Model file for the job. Use its own axes, mm. Round coordinates to 2 decimals unless told otherwise and drop trailing zeros. Loops run counter-clockwise (first coordinate to the right, second up) from the corner with the lowest first, then second, coordinate; pieces in that order, holes last. Notation, with made-up numbers: (33, -18) -> (50, -18) arc R26 ccw to (50, 9) -> close; hole circle Ø10 at (38, 4). An arc over 180 degrees is marked (long way). Use a Markdown table: item, result. Add a question column.
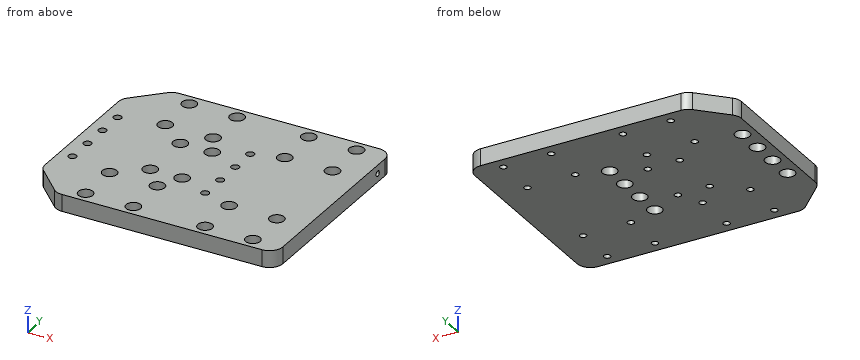
```python
from build123d import *

# Parameters (mm, degrees)
SKETCH1_R                 = 2.5
BOSS_EXTRUDE1_DEPTH       = 12.7
SKETCH2_R                 = 5.5
CUT_EXTRUDE1_DEPTH        = 7
CUT_EXTRUDE2_REACH        = 133.416
SKETCH3_R                 = 3
SKETCH4_R                 = 5.5
CUT_EXTRUDE3_DEPTH        = 7
CHAMFER1_SIZE             = 25
FILLET1_R                 = 10
M5X0_8_TAPPED_HOLE1_D     = 4.2
M5X0_8_TAPPED_HOLE1_DEPTH = 19
M5X0_8_TAPPED_HOLE1_TIP   = 1.2618073


with BuildPart() as part:
    # Sketch1 → Boss-Extrude1 (new body)
    with BuildSketch(Plane.XY):
        Polygon((-85, 78), (85, 78), (85, -78), (-85, -78), (-105, -78), (-105, 78), align=None)
        with Locations((27, -37)):
            Circle(SKETCH1_R, mode=Mode.SUBTRACT)
        with Locations((63, -37)):
            Circle(SKETCH1_R, mode=Mode.SUBTRACT)
        with Locations((27, -69)):
            Circle(SKETCH1_R, mode=Mode.SUBTRACT)
        with Locations((63, -69)):
            Circle(SKETCH1_R, mode=Mode.SUBTRACT)
        with Locations(Location((-63, -37, 0), (0, 0, 180))):
            Circle(SKETCH1_R, mode=Mode.SUBTRACT)
        with Locations(Location((-63, -69, 0), (0, 0, 180))):
            Circle(SKETCH1_R, mode=Mode.SUBTRACT)
        with Locations(Location((-27, -69, 0), (0, 0, 180))):
            Circle(SKETCH1_R, mode=Mode.SUBTRACT)
        with Locations(Location((-27, -37, 0), (0, 0, 180))):
            Circle(SKETCH1_R, mode=Mode.SUBTRACT)
        with Locations(Location((63, 69, 0), (0, 0, 180))):
            Circle(SKETCH1_R, mode=Mode.SUBTRACT)
        with Locations(Location((63, 37, 0), (0, 0, 180))):
            Circle(SKETCH1_R, mode=Mode.SUBTRACT)
        with Locations(Location((27, 69, 0), (0, 0, 180))):
            Circle(SKETCH1_R, mode=Mode.SUBTRACT)
        with Locations(Location((27, 37, 0), (0, 0, 180))):
            Circle(SKETCH1_R, mode=Mode.SUBTRACT)
        with Locations((-27, 69)):
            Circle(SKETCH1_R, mode=Mode.SUBTRACT)
        with Locations((-27, 37)):
            Circle(SKETCH1_R, mode=Mode.SUBTRACT)
        with Locations((-63, 69)):
            Circle(SKETCH1_R, mode=Mode.SUBTRACT)
        with Locations((-63, 37)):
            Circle(SKETCH1_R, mode=Mode.SUBTRACT)
        with Locations((-42, 20)):
            Circle(SKETCH1_R, mode=Mode.SUBTRACT)
        with Locations((-18, 20)):
            Circle(SKETCH1_R, mode=Mode.SUBTRACT)
        with Locations((-42, -20)):
            Circle(SKETCH1_R, mode=Mode.SUBTRACT)
        with Locations((-18, -20)):
            Circle(SKETCH1_R, mode=Mode.SUBTRACT)
    extrude(amount=BOSS_EXTRUDE1_DEPTH)

    # Sketch2 → Cut-Extrude1 (cut)
    with BuildSketch(Plane.XY.offset(12.7)):
        with Locations((-63, 69)):
            Circle(SKETCH2_R)
        with Locations((-27, 69)):
            Circle(SKETCH2_R)
        with Locations((-63, 37)):
            Circle(SKETCH2_R)
        with Locations((-27, 37)):
            Circle(SKETCH2_R)
        with Locations((27, 69)):
            Circle(SKETCH2_R)
        with Locations((63, 69)):
            Circle(SKETCH2_R)
        with Locations((27, 37)):
            Circle(SKETCH2_R)
        with Locations((63, 37)):
            Circle(SKETCH2_R)
        with Locations((-42, 20)):
            Circle(SKETCH2_R)
        with Locations((-18, 20)):
            Circle(SKETCH2_R)
        with Locations((-42, -20)):
            Circle(SKETCH2_R)
        with Locations((-18, -20)):
            Circle(SKETCH2_R)
        with Locations((-63, -37)):
            Circle(SKETCH2_R)
        with Locations((-27, -37)):
            Circle(SKETCH2_R)
        with Locations((-63, -69)):
            Circle(SKETCH2_R)
        with Locations((-27, -69)):
            Circle(SKETCH2_R)
        with Locations((27, -69)):
            Circle(SKETCH2_R)
        with Locations((27, -37)):
            Circle(SKETCH2_R)
        with Locations((63, -37)):
            Circle(SKETCH2_R)
        with Locations((63, -69)):
            Circle(SKETCH2_R)
    extrude(amount=-CUT_EXTRUDE1_DEPTH, mode=Mode.SUBTRACT)

    # Sketch3 → Cut-Extrude2 (cut, up to next)
    with BuildSketch(Plane.XY.offset(12.7), mode=Mode.PRIVATE) as cut_extrude2_sk1:
        with Locations((-95, 30)):
            Circle(SKETCH3_R)
    cut_extrude2_tool1 = extrude(cut_extrude2_sk1.sketch, amount=-CUT_EXTRUDE2_REACH, mode=Mode.PRIVATE) & part.part
    # Sketch3 → Cut-Extrude2 (cut, up to next)
    with BuildSketch(Plane.XY.offset(12.7), mode=Mode.PRIVATE) as cut_extrude2_sk2:
        with Locations((-95, 10)):
            Circle(SKETCH3_R)
    cut_extrude2_tool2 = extrude(cut_extrude2_sk2.sketch, amount=-CUT_EXTRUDE2_REACH, mode=Mode.PRIVATE) & part.part
    # Sketch3 → Cut-Extrude2 (cut, up to next)
    with BuildSketch(Plane.XY.offset(12.7), mode=Mode.PRIVATE) as cut_extrude2_sk3:
        with Locations((-95, -10)):
            Circle(SKETCH3_R)
    cut_extrude2_tool3 = extrude(cut_extrude2_sk3.sketch, amount=-CUT_EXTRUDE2_REACH, mode=Mode.PRIVATE) & part.part
    # Sketch3 → Cut-Extrude2 (cut, up to next)
    with BuildSketch(Plane.XY.offset(12.7), mode=Mode.PRIVATE) as cut_extrude2_sk4:
        with Locations((-95, -30)):
            Circle(SKETCH3_R)
    cut_extrude2_tool4 = extrude(cut_extrude2_sk4.sketch, amount=-CUT_EXTRUDE2_REACH, mode=Mode.PRIVATE) & part.part
    # Sketch3 → Cut-Extrude2 (cut, up to next)
    with BuildSketch(Plane.XY.offset(12.7), mode=Mode.PRIVATE) as cut_extrude2_sk5:
        with Locations((5, -30)):
            Circle(SKETCH3_R)
    cut_extrude2_tool5 = extrude(cut_extrude2_sk5.sketch, amount=-CUT_EXTRUDE2_REACH, mode=Mode.PRIVATE) & part.part
    # Sketch3 → Cut-Extrude2 (cut, up to next)
    with BuildSketch(Plane.XY.offset(12.7), mode=Mode.PRIVATE) as cut_extrude2_sk6:
        with Locations((5, -10)):
            Circle(SKETCH3_R)
    cut_extrude2_tool6 = extrude(cut_extrude2_sk6.sketch, amount=-CUT_EXTRUDE2_REACH, mode=Mode.PRIVATE) & part.part
    # Sketch3 → Cut-Extrude2 (cut, up to next)
    with BuildSketch(Plane.XY.offset(12.7), mode=Mode.PRIVATE) as cut_extrude2_sk7:
        with Locations((5, 10)):
            Circle(SKETCH3_R)
    cut_extrude2_tool7 = extrude(cut_extrude2_sk7.sketch, amount=-CUT_EXTRUDE2_REACH, mode=Mode.PRIVATE) & part.part
    # Sketch3 → Cut-Extrude2 (cut, up to next)
    with BuildSketch(Plane.XY.offset(12.7), mode=Mode.PRIVATE) as cut_extrude2_sk8:
        with Locations((5, 30)):
            Circle(SKETCH3_R)
    cut_extrude2_tool8 = extrude(cut_extrude2_sk8.sketch, amount=-CUT_EXTRUDE2_REACH, mode=Mode.PRIVATE) & part.part
    add(cut_extrude2_tool1.solids().sort_by_distance((-95, 30, 12.7))[0], mode=Mode.SUBTRACT)
    add(cut_extrude2_tool2.solids().sort_by_distance((-95, 10, 12.7))[0], mode=Mode.SUBTRACT)
    add(cut_extrude2_tool3.solids().sort_by_distance((-95, -10, 12.7))[0], mode=Mode.SUBTRACT)
    add(cut_extrude2_tool4.solids().sort_by_distance((-95, -30, 12.7))[0], mode=Mode.SUBTRACT)
    add(cut_extrude2_tool5.solids().sort_by_distance((5, -30, 12.7))[0], mode=Mode.SUBTRACT)
    add(cut_extrude2_tool6.solids().sort_by_distance((5, -10, 12.7))[0], mode=Mode.SUBTRACT)
    add(cut_extrude2_tool7.solids().sort_by_distance((5, 10, 12.7))[0], mode=Mode.SUBTRACT)
    add(cut_extrude2_tool8.solids().sort_by_distance((5, 30, 12.7))[0], mode=Mode.SUBTRACT)

    # Sketch4 → Cut-Extrude3 (cut)
    with BuildSketch(Plane(origin=(0, 0, 0), x_dir=(-1, 0, 0), z_dir=(0, 0, -1))):
        with Locations((-5, 30)):
            Circle(SKETCH4_R)
        with Locations((-5, 10)):
            Circle(SKETCH4_R)
        with Locations((-5, -10)):
            Circle(SKETCH4_R)
        with Locations((-5, -30)):
            Circle(SKETCH4_R)
        with Locations((95, 30)):
            Circle(SKETCH4_R)
        with Locations((95, 10)):
            Circle(SKETCH4_R)
        with Locations((95, -10)):
            Circle(SKETCH4_R)
        with Locations((95, -30)):
            Circle(SKETCH4_R)
    extrude(amount=-CUT_EXTRUDE3_DEPTH, mode=Mode.SUBTRACT)

    # Chamfer1
    chamfer1_edges = [part.edges().sort_by_distance(p)[0] for p in [
        (-105, -78, 6.35),
        (-105, 78, 6.35),
    ]]
    chamfer(chamfer1_edges, length=CHAMFER1_SIZE)

    # Fillet1
    fillet1_edges = [part.edges().sort_by_distance(p)[0] for p in [
        (85, 78, 6.35),
        (85, -78, 6.35),
        (-105, -53, 6.35),
        (-105, 53, 6.35),
        (-80, 78, 6.35),
        (-80, -78, 6.35),
    ]]
    fillet(fillet1_edges, radius=FILLET1_R)

    # M5x0.8 Tapped Hole1
    with Locations(Plane(origin=(85, 0, 0), x_dir=(0, 0, -1), z_dir=(1, 0, 0))):
        with Locations((-6.35, 58.25)):
            Hole(M5X0_8_TAPPED_HOLE1_D / 2, depth=M5X0_8_TAPPED_HOLE1_DEPTH)
            with Locations((0, 0, -(M5X0_8_TAPPED_HOLE1_DEPTH + M5X0_8_TAPPED_HOLE1_TIP / 2))):  # 118° drill point
                Cone(0, M5X0_8_TAPPED_HOLE1_D / 2, M5X0_8_TAPPED_HOLE1_TIP, mode=Mode.SUBTRACT)


solid = part.part
```
1) Pin check, flat tips, straight feed: pin 1 Ø6.5 at (y, z) = (58.25, 6.35) entering from -X; pin 2 Ø5.5 at (x, y) = (-63.5, 68) entering from +Z; pin 3 Ø5 at (x, z) = (-78.5, 6.5) entering from -Y. Stop position of each tip, or through.
2) Cut at B-B on y = 20. Write the cut outline in (x, z).
3) Wall check: probe 1 along Y at (x, z) = (-63, 4.15); probe 2 along X at (y, z) = (37, 2); probe 3 along Y at (x, z) = (-18, 10). Give the ranges that are in metal, low to high. Write a range as from..to.
4) Cut at C-C on x = 5. Count the separate pieces of the cut face and the enclosed holes in it, and give its area (3 significant figures).
5) Cut at A-A on x = -42. Write the cut outline in (y, z).
Established:
| question | item | result |
|---|---|---|
| 1 | pin 1 | stops at x = -102.89 |
| 1 | pin 2 | stops at z = 5.7 |
| 1 | pin 3 | stops at y = -78 |
| 2 | outline | (-105, 0) -> (-44.5, 0) -> (-44.5, 5.7) -> (-47.5, 5.7) -> (-47.5, 12.7) -> (-105, 12.7) -> close; (-39.5, 0) -> (-20.5, 0) -> (-20.5, 5.7) -> (-23.5, 5.7) -> (-23.5, 12.7) -> (-36.5, 12.7) -> (-36.5, 5.7) -> (-39.5, 5.7) -> close; (-15.5, 0) -> (85, 0) -> (85, 12.7) -> (-12.5, 12.7) -> (-12.5, 5.7) -> (-15.5, 5.7) -> close |
| 3 | probe 1 | y = -78..-71.5, -66.5..-39.5, -34.5..34.5, 39.5..66.5, 71.5..78 |
| 3 | probe 2 | x = -105..-65.5, -60.5..-29.5, -24.5..24.5, 29.5..60.5, 65.5..85 |
| 3 | probe 3 | y = -78..-25.5, -14.5..14.5, 25.5..78 |
| 4 | separate pieces | 5 |
| 4 | enclosed holes | 0 |
| 4 | area | 1,540 mm^2 |
| 5 | outline | (-78, 0) -> (-22.5, 0) -> (-22.5, 5.7) -> (-25.5, 5.7) -> (-25.5, 12.7) -> (-78, 12.7) -> close; (-17.5, 0) -> (17.5, 0) -> (17.5, 5.7) -> (14.5, 5.7) -> (14.5, 12.7) -> (-14.5, 12.7) -> (-14.5, 5.7) -> (-17.5, 5.7) -> close; (22.5, 0) -> (78, 0) -> (78, 12.7) -> (25.5, 12.7) -> (25.5, 5.7) -> (22.5, 5.7) -> close |
